Geometry: final body of the model. Coordinates: model frame, mm. A direction names the side the tool comes from. Give positions to 0.01 mm unless a question says otherwise; leave off trailing zeros. Write each loop counter-clockwise with the first axis right and the second up, starting at its lowest first coordinate (ties: lowest second). Pieces come first, ordered by that corner, then holes. Notation, with made-up numbers: (0.25, 81) -> (41.25, 81) arc R15 ccw to (41.25, 109) -> close; hole circle Ø4 at (51, 62). An arc over 180 degrees is marked (long way). Answer as a JSON object with one key per item and string values.
Autodesk Inventor part; units mm, degrees
ref_plane "YZ Plane" through (0, 0, 0) normal (1, 0, 0) x (0, 1, 0)
ref_plane "XZ Plane" through (0, 0, 0) normal (0, 1, 0) x (-1, 0, 0)
ref_plane "XY Plane" through (0, 0, 0) normal (0, 0, 1) x (1, 0, 0)
sketch "Sketch1" plane through (0, 0, 0) normal (0, 1, 0) x (-1, 0, 0)
  line L0 (44.8336, -32.5735) -> (17.1249, -52.705)
  line L1 (17.1249, -52.705) -> (-17.1249, -52.705)
  line L2 (-17.1249, -52.705) -> (-44.8336, -32.5735)
  line L3 (48.4634, -35.2108) -> (18.5114, -56.9722)
  line L4 (18.5114, -56.9722) -> (-18.5114, -56.9722)
  line L5 (-18.5114, -56.9722) -> (-48.4634, -35.2108)
  line L6 (48.4634, -35.2108) -> (44.8336, -32.5735)
  line L7 (-44.8336, -32.5735) -> (-48.4634, -35.2108)
  point P0 (0, 0)
  point P1 (0, 0)
  point P2 (0, 0)
  dimension "d0" = 52.705
  dimension "d1" = 4.2672
extrude "Extrusion1" add sketch "Sketch1" along normal blind 76.2
sketch "Sketch2" plane through (18.5114, 0, -56.9722) normal (0.5878, 0, -0.809) x (-0.809, 0, -0.5878)
  circle A0 centre (-18.5114, 38.1) radius 2.921
  line L0 (-37.0228, 76.2) -> (0, 76.2)
  point P0 (-18.5114, 0)
  dimension "d4" = 5.842
  dimension "d5" = 38.1
sketch "Sketch3" plane through (18.5114, 0, -56.9722) normal (0, 0, -1) x (-1, 0, 0)
  circle A0 centre (18.5114, 38.1) radius 2.921
  line L0 (0, 76.2) -> (37.0228, 76.2)
  point P0 (18.5114, 0)
  dimension "d6" = 5.842
  dimension "d7" = 38.1
sketch "Sketch4" plane through (-48.4634, 0, -35.2108) normal (-0.5878, 0, -0.809) x (-0.809, 0, 0.5878)
  circle A0 centre (-18.5114, 38.1) radius 2.921
  line L0 (-37.0228, 76.2) -> (0, 76.2)
  point P0 (-18.5114, 0)
  dimension "d8" = 5.842
  dimension "d9" = 38.1
extrude "Extrusion2" cut sketch "Sketch2" against normal through all
extrude "Extrusion3" cut sketch "Sketch3" against normal blind 4.2672
extrude "Extrusion4" cut sketch "Sketch4" against normal blind 4.2672
sketch "Sketch5" plane through (18.5114, 0, -56.9722) normal (0, 0, -1) x (-1, 0, 0)
  circle A0 centre (18.5114, 38.1) radius 2.921
  circle A1 centre (18.5114, 47.5742) radius 2.921
  circle A2 centre (11.8121, 44.7993) radius 2.921
  circle A3 centre (9.0372, 38.1) radius 2.921
  circle A4 centre (11.8121, 31.4007) radius 2.921
  circle A5 centre (18.5114, 28.6258) radius 2.921
  circle A6 centre (25.2107, 31.4007) radius 2.921
  circle A7 centre (27.9856, 38.1) radius 2.921
  circle A8 centre (25.2107, 44.7993) radius 2.921
  point P0 (18.5114, 0)
  dimension "d17" = 5.842
  dimension "d21" = 360
extrude "Extrusion5" cut sketch "Sketch5" against normal through all contours A1 | A2 | A3 | A4 | A5 | A6 | A7 | A8
properties part number "10 bracket"
Q1. Set-up query: faces 1 (the cylindrical face through (7.08, 47.695, -54.868)), 2 (the flat face through (-4, 38, -52.705)). Return all of +Z, -Z, +X, -X, +Y, -Y with unobstructed straight access to the full face (end or side cutting, diameter ignored); none if empty.
Values:
{"face 1": "+Z, -Z", "face 2": "+Z, +Y, -Y"}
Q2. First-contact query: P1, Ø17, axis at x = -1.5, y = 42, coming from the +Z side (3 decimals); P2, Ø4.5, axis at x = 0, y = 47.57, coming from the +Z side; P3, Ø4, axis at y = 11, z = -44, coming from the +X side; P4, Ø4, axis at y = 57, z = -48.5, coming from the +X side. Flat tips, straight axial feed; report the tip coordinate or a pass-through.
Values:
{"P1": "z = -52.705", "P2": "through", "P3": "x = 39.12", "P4": "x = 32.93"}
Q3. Mould query, pull axis Y, two halves, no side actions, for faces 3 (the cylindrical face through (31.16, 35.51, -45.18)), 4 (the flat face through (46.62, 37.57, -33.87)), 5 (the flat face through (0, 76.2, -53)). Classes: pulls with the +Y half, pulls with the -Y half, needs draft (parallel to the pull), parting line crosses it, or undercut.
Values:
{"face 3": "undercut", "face 4": "needs draft", "face 5": "pulls with the +Y half"}
Q4. Cut plane D-D (y = 49). Return the cut outline in (x, z) (1 decimal).
Values:
{"outline": "(-48.5, -35.2) -> (-18.5, -57) -> (-2.5, -57) -> (-2.5, -52.7) -> (-17.1, -52.7) -> (-44.8, -32.6) -> close; (2.5, -57) -> (18.5, -57) -> (48.5, -35.2) -> (44.8, -32.6) -> (17.1, -52.7) -> (2.5, -52.7) -> close"}
Q5. Cut plane C-C (y = 38.1). Return the cut outline in (x, z) (1 decimal).
Values:
{"outline": "(-48.5, -35.2) -> (-35.9, -44.4) -> (-33.3, -40.9) -> (-44.8, -32.6) -> close; (-31.1, -47.8) -> (-18.5, -57) -> (-12.4, -57) -> (-12.4, -52.7) -> (-17.1, -52.7) -> (-28.6, -44.4) -> close; (-6.6, -57) -> (-2.9, -57) -> (-2.9, -52.7) -> (-6.6, -52.7) -> close; (2.9, -57) -> (6.6, -57) -> (6.6, -52.7) -> (2.9, -52.7) -> close; (12.4, -57) -> (18.5, -57) -> (31.1, -47.8) -> (28.6, -44.4) -> (17.1, -52.7) -> (12.4, -52.7) -> close; (33.3, -40.9) -> (35.9, -44.4) -> (48.5, -35.2) -> (44.8, -32.6) -> close"}
Q6. Material intervals for L1, parallel to Y at x = 0, z = -55.8; L2, parallel to Z at x = -9, y = 24 (3 decimals); L3, parallel to X at y = 21.5, z = -40.75, sorted ascending. Write a range as from..to.
Values:
{"L1": "0..25.7, 31.55..35.18, 41.02..44.65, 50.5..76.2", "L2": "-56.972..-52.705", "L3": "-40.84..-33.58, 33.58..40.84"}
Q7. Cut plane A-A (x = 0). Return the cut outline in (y, z) (3 decimals), and give its area (3 significant figures).
Values:
{"outline": "(0, -56.972) -> (25.705, -56.972) -> (25.705, -52.705) -> (0, -52.705) -> close; (31.547, -56.972) -> (35.179, -56.972) -> (35.179, -52.705) -> (31.547, -52.705) -> close; (41.021, -56.972) -> (44.653, -56.972) -> (44.653, -52.705) -> (41.021, -52.705) -> close; (50.495, -56.972) -> (76.2, -56.972) -> (76.2, -52.705) -> (50.495, -52.705) -> close", "area": "250 mm²"}
Q8. Cut plane B-B (z = -49.25). Return the cut outline in (x, y), and give its area (3 significant figures).
Values:
{"outline": "(-29.14, 0) -> (-21.88, 0) -> (-21.88, 76.2) -> (-29.14, 76.2) -> close; (21.88, 0) -> (29.14, 0) -> (29.14, 76.2) -> (21.88, 76.2) -> close", "area": "1,110 mm²"}
